Design review of the part built by this model. Coordinates are the model's own, in mm. A direction names the side the tool comes from. Coordinates: 2 decimals unless noted, no trailing zeros. Order: outer loops, then holes, each group sorted by start corner. A loop starts at its lowest first (then second) coordinate and runs counter-clockwise, first axis right, second up. Notation, with made-up numbers: (34.25, 50.25) - (93.25, 50.25) arc R10 cw to (93.25, 65.25) - close; hole circle Ø1 at (84.5, 70). An arc over 180 degrees is marked (long way). Write item = value, one per line. Start each with the question number.
```python
from build123d import *

# Parameters (mm, degrees)
F1_DEPTH = 4
F2_COUNT = 9
F4_R     = 1.5
F5_DEPTH = 4


with BuildPart() as f1:
    # F0 (on Top) → F1 (new body)
    with BuildSketch(Plane.XY):
        with BuildLine():
            Line((8.305078, 3.467805), (0, 0))
            Line((0, 0), (8.305078, -3.467805))
            ThreePointArc((8.305078, -3.467805), (8.464361, -3.058527), (8.603489, -2.641966))
            ThreePointArc((8.603489, -2.641966), (9.047406, -2.076548), (9.755918, -1.955011))
            Line((9.755918, -1.955011), (9.805066, -1.96486))
            ThreePointArc((9.805066, -1.96486), (11.163417, -2.001728), (12.455768, -1.581844))
            ThreePointArc((12.455768, -1.581844), (12.819329, -1.255462), (12.98487, -0.795791))
            Line((12.98487, -0.795791), (13.06382, 0))
            Line((13.06382, 0), (12.98487, 0.795791))
            ThreePointArc((12.98487, 0.795791), (12.819329, 1.255462), (12.455768, 1.581844))
            ThreePointArc((12.455768, 1.581844), (11.163417, 2.001728), (9.805066, 1.96486))
            Line((9.805066, 1.96486), (9.755918, 1.955011))
            ThreePointArc((9.755918, 1.955011), (9.047406, 2.076548), (8.603489, 2.641966))
            ThreePointArc((8.603489, 2.641966), (8.464361, 3.058527), (8.305078, 3.467805))
        make_face()
    extrude(amount=F1_DEPTH)


with BuildPart() as f2_1:
    # F2: instance of F1
    add(f1.part.rotate(Axis((0, 0, 2), (0, 0, 1)), 1 * 360 / F2_COUNT))


with BuildPart() as f2_2:
    # F2: instance of F1
    add(f1.part.rotate(Axis((0, 0, 2), (0, 0, 1)), 2 * 360 / F2_COUNT))


with BuildPart() as f2_3:
    # F2: instance of F1
    add(f1.part.rotate(Axis((0, 0, 2), (0, 0, 1)), 3 * 360 / F2_COUNT))


with BuildPart() as f2_4:
    # F2: instance of F1
    add(f1.part.rotate(Axis((0, 0, 2), (0, 0, 1)), 4 * 360 / F2_COUNT))


with BuildPart() as f2_5:
    # F2: instance of F1
    add(f1.part.rotate(Axis((0, 0, 2), (0, 0, 1)), 5 * 360 / F2_COUNT))


with BuildPart() as f2_6:
    # F2: instance of F1
    add(f1.part.rotate(Axis((0, 0, 2), (0, 0, 1)), 6 * 360 / F2_COUNT))


with BuildPart() as f2_7:
    # F2: instance of F1
    add(f1.part.rotate(Axis((0, 0, 2), (0, 0, 1)), 7 * 360 / F2_COUNT))


with BuildPart() as f2_8:
    # F2: instance of F1
    add(f1.part.rotate(Axis((0, 0, 2), (0, 0, 1)), 8 * 360 / F2_COUNT))


with BuildPart() as f2_7_1:
    add(f2_7.part)

    # F3: union F2_6, F2_4, F2_5, F1, F2_1, F2_3, F2_2, F2_8
    add(f2_6.part)
    add(f2_4.part)
    add(f2_5.part)
    add(f1.part)
    add(f2_1.part)
    add(f2_3.part)
    add(f2_2.part)
    add(f2_8.part)

    # F4 (on face) → F5 (cut, through all)
    with BuildSketch(Plane.XY.offset(4)):
        Circle(F4_R)
    extrude(amount=-F5_DEPTH, mode=Mode.SUBTRACT)


solid = f2_7_1.part
```
Item 1: Mouldability with a two-part tool opening along X and no side actions: class faces 4 (the cylindrical face through (-5.32, 11.73, 1.97)), 5 (the flat face through (0, 3, 4)), 6 (the cylindrical face through (-0.467, 9.278, 1.972)), 7 (the cylindrical face through (-12.474, -3.198, 1.972)) as +X half, -X half, draft (parallel to the pull), parting line (faces both ways), or undercut.
Item 2: For faces 1 (the cylindrical face through (9.851, -5.657, 1.972)), 2 (the cylindrical face through (-9.8, -5.7, 2)), 3 (the cylindrical face through (-9.22, 1.15, 1.97)), list the 3-axis set-ups (+Z, -Z, +X, -X, +Y, -Y) from which the entire face can be reached by the end or side of a thin tool; tool diameter is ignored.
Item 3: For P1, Ø2, axis at x = 7.5, z = 0.5, coming from the +Y side; P2, Ø1.5, axis at y = 3, z = 2, coming from the +X side; P3, Ø2, axis at x = 4, z = 2, coming from the +Y side, all flat-tipped, find the tip position at first contact; note any pin that passes through.
Item 4: Add section A-A on x = 11.25. Give the boundary of the cut face in (y, z).
Item 5: For line 1 (Y direction, x = -7, z = 2.9); line 2 (Y direction, x = 11.5, z = 1.4); line 3 (Y direction, x = -9.5, z = 1.2), list the stretches that pass through material, from the lowest coordinate up.
Worked out:
q1.face_4 = undercut
q1.face_5 = draft
q1.face_6 = undercut
q1.face_7 = -X half
q2.face_1 = +Z, -Z, +X
q2.face_2 = +Z, -Z, -Y
q2.face_3 = +Z, -Z, -X
q3.P1 = 9.21
q3.P2 = 8.83
q3.P3 = 12.66
q4.outline = (-1.99, 0) - (1.99, 0) - (1.99, 4) - (-1.99, 4) - close
q5.line_1 = -10.98 to -8.04, -5.66 to 5.66, 8.04 to 10.98
q5.line_2 = -1.94 to 1.94
q5.line_3 = -5.62 to -1.38, 1.38 to 5.62
